from build123d import *

# Parameters (mm, degrees)
F0_R     = 20
F1_DEPTH = 150
F2_R     = 15
F2_R_2   = 6
F3_DEPTH = 50
F4_DEPTH = 150
F5_R     = 20
F5_R_2   = 15
F6_DEPTH = 50


with BuildPart() as f1:
    # F0 (on Right) → F1 (new body)
    with BuildSketch(Plane.YZ):
        Circle(F0_R)
    extrude(amount=F1_DEPTH)

    # F2 (on face) → F3 (cut)
    with BuildSketch(Plane(origin=(0, 0, 0), x_dir=(0, -1, 0), z_dir=(-1, 0, 0))):
        Circle(F2_R)
        Circle(F2_R_2, mode=Mode.SUBTRACT)
    extrude(amount=-F3_DEPTH, mode=Mode.SUBTRACT)

    # F4 (cut): a face of the model
    f4_faces = [f1.faces().sort_by_distance(p)[0] for p in [
        (0, 0, 0),
    ]]
    extrude(f4_faces, amount=-F4_DEPTH, mode=Mode.SUBTRACT)

    # F5 (on face) → F6 (cut)
    with BuildSketch(Plane.YZ.offset(150)):
        Circle(F5_R)
        Circle(F5_R_2, mode=Mode.SUBTRACT)
    extrude(amount=-F6_DEPTH, mode=Mode.SUBTRACT)


solid = f1.part
The listing builds one solid part. Answer for the finished solid, in the listing's coordinates (mm). A direction names the side the tool comes from. Coordinates: 2 decimals unless noted, no trailing zeros. Loops run counter-clockwise (first coordinate to the right, second up) from the corner with the lowest first, then second, coordinate; pieces in that order, holes last.
1) Find the intervals of material crossed by L1, parallel to Z at x = 123.5, y = 0; L2, parallel to Z at x = 14.5, y = 0; L3, parallel to Y at x = 27, z = -0.5, in increasing order.
2) A tool of negligible diameter and unlimited length cuts with its end or side. For faces 1 (the face through (125.35, -14.985, 0.66)), 2 (the face through (99, 6, 0)), 3 (the face through (24.65, 14.985, 0.66)), from which of +Z, -Z, +X, -X, +Y, -Y can it reach the whole face along a straight path? Write none if from no direction.
3) Flat-ended cylindrical pins translate along their axes: pin 1 Ø6 at (x, z) = (81, 3.5) entering from -Y; pin 2 Ø15 at (y, z) = (-6, 2) entering from -X; pin 3 Ø5 at (x, y) = (57, 3.5) entering from -Z (3 decimals). Find the tip coordinate at first contact, or state that the pin passes through.
4) Find section D-D on z = -8. Write down the section's boundary in (x, y), then the cut area to 3 significant figures.
5) Find section A-A on z = 0. Write down the section's boundary in (x, y), then the cut area to 3 significant figures.
6) Determine the mould class of faces 4 (the face through (0, 3, 15)), 5 (the face through (50, -6.5, 0.2)), 6 (the face through (49.3, -4.336, -19.524)) for opening direction Y: pulls with the +Y half, pulls with the -Y half, needs draft (parallel to the pull), parting line crosses it, or undercut.
7) Find section C-C on x = 127. Write down the section's boundary in (y, z).
Values:
1. L1: z = -15 to -6, 6 to 15
1. L2: z = -20 to -15, 15 to 20
1. L3: y = -19.99 to -14.99, 14.99 to 19.99
2. face 1: +X
2. face 2: +X, -X
2. face 3: -X
3. pin 1: stops at y = -19.99
3. pin 2: stops at x = 50
3. pin 3: stops at z = -19.975
4. outline: (0, -18.33) - (100, -18.33) - (100, -12.69) - (150, -12.69) - (150, 12.69) - (100, 12.69) - (100, 18.33) - (0, 18.33) - (0, 12.69) - (50, 12.69) - (50, -12.69) - (0, -12.69) - close
4. area: 3,670 mm2
5. outline: (0, -20) - (100, -20) - (100, -15) - (150, -15) - (150, -6) - (50, -6) - (50, -15) - (0, -15) - close; (0, 15) - (50, 15) - (50, 6) - (150, 6) - (150, 15) - (100, 15) - (100, 20) - (0, 20) - close
5. area: 2,800 mm2
6. face 4: needs draft
6. face 5: undercut
6. face 6: parting line crosses it
7. outline: circle Ø30 at (0, 0); hole circle Ø12 at (0, 0)
